Input: part model. Units: mm. Frame: model coordinates. A direction names the side the tool comes from. Round coordinates to 2 decimals unless told otherwise and drop trailing zeros. Loops run counter-clockwise (first coordinate to the right, second up) from the corner with the lowest first, then second, coordinate; pieces in that order, holes last. Notation, with made-up numbers: (34.25, 22.25) - (73.25, 22.25) arc R23 cw to (73.25, 40.25) - close; hole circle Ø9 at (45, -5). An arc over 180 degrees is marked (long way). Use CSV: the item, a comma, the result in double quotes. Start each with the question number.
1. Pull-direction query (Z, two-part tool) for faces 1 (the flat face through (-1, 8.5, -1)), 2 (the flat face through (1, 8, 0.4)), 3 (the cylindrical face through (0.54, 6.86, -2.44)); classes: +Z half, -Z half, draft (parallel to the pull), parting line (faces both ways), or undercut.
2. Pin query (flat end, axial travel): P1, Ø1, axis at x = -1, y = 6, coming from the -Z side; P2, Ø1.2, axis at y = 8, z = 1, coming from the +X side; P3, Ø1.2, axis at x = -1.5, y = 7.5, coming from the -Z side. Return the tip coordinate at first contact, or that it passes through.
3. Material intervals for probe 1 along Y at (x, z) = (1.3, 0.3); probe 2 along Y at (x, z) = (0, 1.85); probe 3 along Z at (x, y) = (-0.95, 7.5), sorted ascending. Write a range as from..to.
4. Cut plane C-C (y = 3.5). Return loops of the section in (x, z), and give its area (3 significant figures).
5. Cut plane B-B (z = 0). Return loops of the section in (x, y).
6. Access query for faces 4 (the flat face through (0, 0, 0)), 5 (the cylindrical face through (1.5, 3.04, 0.07)), 6 (the flat face through (2, 8, 0)). Directions: +Z, -Z, +X, -X, +Y, -Y. A direction counts if a zero-diameter tool reaches every point of the face in a straight line with its end or side. Return the directions, or none.
7. Cut plane A-A (x = 0). Return loops of the section in (y, z).
```python
from build123d import *

# Parameters (mm, degrees)
REDONDEO1_R           = 0.8
CORTAR_EXTRUIR1_DEPTH = 1.5


with BuildPart() as part:
    # Croquis1 → Revolución1 (revolve)
    with BuildSketch(Plane.XY):
        Polygon((0, 0), (-1.5, 0), (-1.5, 6), (-2.5, 6), (-2.5, 8.5), (0, 8.5), align=None)
    revolve(axis=Axis((0, 0, 0), (0, 1, 0)))

    # Redondeo1
    redondeo1_edges = [part.edges().sort_by_distance(p)[0] for p in [
        (2.5, 8.5, 0),
    ]]
    fillet(redondeo1_edges, radius=REDONDEO1_R)

    # Croquis2 → Cortar-Extruir1 (cut)
    with BuildSketch(Plane(origin=(0, 8.5, 0), x_dir=(1, 0, 0), z_dir=(0, 1, 0))):
        Polygon((0.4, -2), (0.4, -0.4), (2, -0.4), (2, 0.4), (0.4, 0.4), (0.4, 2), (-0.4, 2), (-0.4, 0.4), (-2, 0.4), (-2, -0.4), (-0.4, -0.4), (-0.4, -2), align=None)
    extrude(amount=-CORTAR_EXTRUIR1_DEPTH, mode=Mode.SUBTRACT)


solid = part.part
```
Established:
1,face 1,"draft"
1,face 2,"undercut"
1,face 3,"parting line"
2,P1,"stops at z = -2.45"
2,P2,"stops at x = 2.46"
2,P3,"stops at z = -2.33"
3,probe 1,"y = 0..7"
3,probe 2,"y = 6..7"
3,probe 3,"z = -2.31..-0.4, 0.4..2.31"
4,outline,"circle Ø3 at (0, 0)"
4,area,"7.07 mm2"
5,outline,"(-2.5, 6) - (-1.5, 6) - (-1.5, 0) - (1.5, 0) - (1.5, 6) - (2.5, 6) - (2.5, 7.7) arc R0.8 ccw to (2, 8.44) - (2, 7) - (-2, 7) - (-2, 8.44) arc R0.8 ccw to (-2.5, 7.7) - close"
6,face 4,"+Z, -Z, +X, -X, -Y"
6,face 5,"-Y"
6,face 6,"+Y"
7,outline,"(0, -1.5) - (6, -1.5) - (6, -2.5) - (7.7, -2.5) arc R0.8 ccw to (8.44, -2) - (7, -2) - (7, 2) - (8.44, 2) arc R0.8 ccw to (7.7, 2.5) - (6, 2.5) - (6, 1.5) - (0, 1.5) - close"
